Geometry check sheet. Reference: the model listing, model coordinates, mm. A direction names the side the tool comes from. Give positions to 0.01 mm unless a question says otherwise; leave off trailing zeros. Loops run counter-clockwise (first coordinate to the right, second up) from the corner with the lowest first, then second, coordinate; pieces in that order, holes last. Notation, with made-up numbers: (-19.75, 12) -> (-0.75, 12) arc R13 ccw to (-0.75, 36) -> close; hole circle Ø10 at (-1.75, -40). An arc over 180 degrees is marked (long way). Write each question's results on one line, items separated by ' | '. Start each with the question number.
1) Scan lines: line 1 (Z direction, x = 0, y = 1); line 2 (X direction, y = 0.25, z = -97); line 3 (Y direction, x = 0, z = -4). Record each from-to range of solid material in increasing order. Write a range as from..to.
2) Set-up check for faces 5 (the face through (0.59, 4.46, -34.26)), 6 (the face through (0, 0, -10)), 7 (the face through (0, 0, -100)): record each of +Z, -Z, +X, -X, +Y, -Y from which the full face is reachable in a straight line by a thin tool's end or side.
3) Sectioned sample at B-B on y = 0. Record the cut outline in (x, z).
4) Depth check by flat-ended pin: pin 1 (6 mm diameter, centred on x = -3.5, z = -16, fed in from +Y); pin 2 (2 mm diameter, centred on x = -2, z = -28.5, fed in from +Y); pin 3 (1.5 mm diameter, centred on x = -0.5, y = 0.5, fed in from +Z). Enter the tip coordinate at first touch or a pass-through.
5) Sectioned sample at A-A on x = 0. Record the cut outline in (y, z).
6) Sectioned sample at C-C on z = -97. Record the cut outline in (x, y).
7) Draft check along X on faces 1 (the face through (1.08, -4.88, -17.48)), 2 (the face through (0.38, 0.07, -98.71)), 3 (the face through (-2, 0, 0)), 4 (the face through (-1.5, 0.07, -4.93)). Enter one of: pulls with the +X half, pulls with the -X half, needs draft (parallel to the pull), parting line crosses it, or undercut.
8) Sectioned sample at D-D on z = -20. Record the cut outline in (x, y), then the cut area to 3 significant figures.
Autodesk Inventor part; units mm, degrees
ref_plane "Work Plane1" through (0, 5, -67.0015) normal (0, 1, 0) x (-1, 0, 0)
ref_plane "YZ Plane" through (0, 0, 0) normal (1, 0, 0) x (0, 1, 0)
ref_plane "XY Plane" through (0, 0, 0) normal (0, 0, 1) x (1, 0, 0)
sketch "Sketch1" plane through (0, 0, 0) normal (0, 1, 0) x (-1, 0, 0)
  line L0 (0, 0) -> (5, 0)
  line L1 (5, 0) -> (5, -100)
  line L2 (5, -100) -> (0, -100)
  line L3 (0, -100) -> (0, 0)
  line L4 (5, -33.5) -> (4.5, -33.5)
  line L5 (4.5, -33.5) -> (4.5, -35)
  line L6 (4.5, -35) -> (5, -35)
  line L7 (5, -35) -> (5, -33.5)
  line L8 (5, -90) -> (0, -90) construction
  line L9 (5, -99.003) -> (4.003, -100)
  line L10 (4, 0) -> (5, -1)
  dimension "d0" = 5
  dimension "d1" = 100
  dimension "d2" = 1.5
  dimension "d3" = 0.5
  dimension "d4" = 135
  dimension "d5" = 10
  dimension "d6" = 55
  dimension "d7" = 1.41
  dimension "d8" = 45
  dimension "d9" = 1.4142
revolve "Revolution1" add sketch "Sketch1" angle 360 about axis through (0, 0, -100) along (0, 0, 1) contours L0 L10 L1 L4 L5 L6 L9 L2 L3
ref_plane "Work Plane1" through (0, 5, -67.0015) normal (0, 1, 0) x (-1, 0, 0)
sketch "Sketch2" plane through (0, 5, -67.0015) normal (0, 1, 0) x (-1, 0, 0)
  circle A0 centre (0, -29.9985) radius 1.75
  line L0 (-4.003, -32.9985) -> (4.003, -32.9985)
  point P0 (0, 67.0015)
  dimension "d11" = 3.5
  dimension "d12" = 3
extrude "Extrusion1" cut sketch "Sketch2" against normal blind 10
sketch "Sketch3" plane through (0, 0, 0) normal (0, 0, 1) x (1, 0, 0)
  circle A0 centre (0, 0) radius 1.5
  dimension "d15" = 3
extrude "Extrusion2" cut sketch "Sketch3" against normal blind 10
thread "Thread1"
properties part number "10mmPins"
Result:
1) line 1: -100..-98.75, -95.25..-10 | line 2: -4.99..-1.75, 1.75..4.99 | line 3: -5..-1.5, 1.5..5
2) face 5: none | face 6: +Z | face 7: -Z, +X, -X, +Y, -Y
3) outline: (-5, -99) -> (-4, -100) -> (4, -100) -> (5, -99) -> (5, -35) -> (4.5, -35) -> (4.5, -33.5) -> (5, -33.5) -> (5, -1) -> (4, 0) -> (1.5, 0) -> (1.5, -10) -> (-1.5, -10) -> (-1.5, 0) -> (-4, 0) -> (-5, -1) -> (-5, -33.5) -> (-4.5, -33.5) -> (-4.5, -35) -> (-5, -35) -> close; hole circle Ø3.5 at (0, -97)
4) pin 1: y = 4.97 | pin 2: y = 4.9 | pin 3: z = -10
5) outline: (-5, -99) -> (-4, -100) -> (4, -100) -> (5, -99) -> (5, -98.75) -> (-5, -98.75) -> close; (-5, -95.25) -> (5, -95.25) -> (5, -35) -> (4.5, -35) -> (4.5, -33.5) -> (5, -33.5) -> (5, -1) -> (4, 0) -> (1.5, 0) -> (1.5, -10) -> (-1.5, -10) -> (-1.5, 0) -> (-4, 0) -> (-5, -1) -> (-5, -33.5) -> (-4.5, -33.5) -> (-4.5, -35) -> (-5, -35) -> close
6) outline: (-1.75, -4.68) -> (-1.75, 4.68) arc R5 ccw to start; (1.75, -4.68) arc R5 ccw to (1.75, 4.68) -> close
7) face 1: parting line crosses it | face 2: undercut | face 3: needs draft | face 4: undercut
8) outline: circle Ø10 at (0, 0) | area: 78.5 mm^2
